Check sheet for the modelled part. Datum: model origin and axes. Units: mm. A direction names the side the tool comes from. Give positions to 0.01 mm unless a question says otherwise; leave off trailing zeros. Write each loop counter-clockwise with the first axis right and the second up, starting at its lowest first coordinate (ties: lowest second). Pieces come first, ordered by that corner, then holes. Notation, with made-up numbers: (-37.75, 50) -> (-14.75, 50) arc R26 cw to (-14.75, 81) -> close; hole circle Ø3 at (-8, 41). An arc over 180 degrees is marked (long way). Answer as a JSON object with one key per item and string values.
from build123d import *

# Parameters (mm, degrees)
BOSS_EXTRU_1_DEPTH                                 = 15
CHAMBRAGE_POUR_VIS_T_TE_HEXAGONALE_M81_D           = 9
CHAMBRAGE_POUR_VIS_T_TE_HEXAGONALE_M81_CBORE_D     = 15
CHAMBRAGE_POUR_VIS_T_TE_HEXAGONALE_M81_CBORE_DEPTH = 8.6
TAP_DRILL_FOR_M5_TAP1_D                            = 4.2
TAP_DRILL_FOR_M5_TAP1_DEPTH                        = 13
TAP_DRILL_FOR_M5_TAP1_TIP                          = 1.2618073
SKETCH25_W                                         = 14
SKETCH25_H                                         = 15
CUT_EXTRUDE6_DEPTH                                 = 16
CONG_1_R                                           = 6
SKETCH11_R                                         = 8.5
CUT_EXTRUDE1_DEPTH                                 = 16
SKETCH12_R                                         = 11
CUT_EXTRUDE2_DEPTH                                 = 11
SKETCH13_W                                         = 24
SKETCH13_H                                         = 24
CUT_EXTRUDE3_DEPTH                                 = 16
FILLET1_R                                          = 6
CUT_EXTRUDE4_DEPTH                                 = 6
FILLET3_R                                          = 14
TAP_DRILL_FOR_M3_TAP1_D                            = 2.5
CHAMFER1_SIZE                                      = 0.5
TAP_DRILL_FOR_M3_TAP2_D                            = 2.5
TAP_DRILL_FOR_M3_TAP3_D                            = 2.5
TROU_POUR_TARAUDAGE_POUR_TROU_TARAUD_M6_D          = 5
TROU_POUR_TARAUDAGE_POUR_TROU_TARAUD_M6_DEPTH      = 20
TROU_POUR_TARAUDAGE_POUR_TROU_TARAUD_M6_TIP        = 1.502151548


with BuildPart() as part:
    # Esquisse1 → Boss.-Extru.1 (new body)
    with BuildSketch(Plane.XY):
        Polygon((-21.072673536, 123.242590707), (54.927326464, 123.242590707), (54.927326464, 18.242590707), (130.927326464, 18.242590707), (130.927326464, -26.757409293), (115.927326464, -26.757409293), (-4.072673536, -146.757409293), (-169.072673536, -146.757409293), (-169.072673536, -76.757409293), (-139.072673536, -46.757409293), (-88.072673536, -46.757409293), (-41.072673536, 0.242590707), (-41.072673536, 103.242590707), align=None)
    extrude(amount=BOSS_EXTRU_1_DEPTH)

    # Chambrage pour vis à tête hexagonale M81 (through all)
    with Locations(Plane(origin=(0, 0, 0), x_dir=(-1, 0, 0), z_dir=(0, 0, -1))):
        with Locations((72.572673536, -78.257409293), (117.572673536, -78.257409293), (72.572673536, -135.257409293), (117.572673536, -135.257409293), (-32.427326464, 85.742590707), (-32.427326464, 40.742590707), (-32.427326464, -4.257409293), (-77.427326464, -4.257409293), (12.572673536, 40.742590707)):
            CounterBoreHole(CHAMBRAGE_POUR_VIS_T_TE_HEXAGONALE_M81_D / 2, CHAMBRAGE_POUR_VIS_T_TE_HEXAGONALE_M81_CBORE_D / 2, CHAMBRAGE_POUR_VIS_T_TE_HEXAGONALE_M81_CBORE_DEPTH)

    # Tap Drill for M5 Tap1
    with Locations(Plane(origin=(0, -146.757409293, 0), x_dir=(-1, 0, 0), z_dir=(0, -1, 0))):
        with Locations((13.072673536, -7.5)):
            Hole(TAP_DRILL_FOR_M5_TAP1_D / 2, depth=TAP_DRILL_FOR_M5_TAP1_DEPTH)
            with Locations((0, 0, -(TAP_DRILL_FOR_M5_TAP1_DEPTH + TAP_DRILL_FOR_M5_TAP1_TIP / 2))):  # 118° drill point
                Cone(0, TAP_DRILL_FOR_M5_TAP1_D / 2, TAP_DRILL_FOR_M5_TAP1_TIP, mode=Mode.SUBTRACT)

    # Sketch25 → Cut-Extrude6 (cut, through all)
    with BuildSketch(Plane(origin=(0, 0, 0), x_dir=(-1, 0, 0), z_dir=(0, 0, -1))):
        with Locations((95.072673536, -54.257409293)):
            Rectangle(SKETCH25_W, SKETCH25_H)
    extrude(amount=-CUT_EXTRUDE6_DEPTH, mode=Mode.SUBTRACT)

    # Congé1
    cong_1_edges = [part.edges().sort_by_distance(p)[0] for p in [
        (-88.072673536, -61.757409293, 7.5),
        (-102.072673536, -46.757409293, 7.5),
        (-102.072673536, -61.757409293, 7.5),
        (54.927326464, 18.242590707, 7.5),
        (130.927326464, 18.242590707, 7.5),
        (130.927326464, -26.757409293, 7.5),
        (115.927326464, -26.757409293, 7.5),
        (-4.072673536, -146.757409293, 7.5),
        (-169.072673536, -76.757409293, 7.5),
        (-139.072673536, -46.757409293, 7.5),
        (-88.072673536, -46.757409293, 7.5),
        (-41.072673536, 0.242590707, 7.5),
        (-41.072673536, 103.242590707, 7.5),
        (-21.072673536, 123.242590707, 7.5),
        (54.927326464, 123.242590707, 7.5),
    ]]
    fillet(cong_1_edges, radius=CONG_1_R)

    # Sketch11 → Cut-Extrude1 (cut, through all)
    with BuildSketch(Plane(origin=(0, 0, 0), x_dir=(-1, 0, 0), z_dir=(0, 0, -1))):
        with Locations((155.072673536, -132.757409293)):
            Circle(SKETCH11_R)
    extrude(amount=-CUT_EXTRUDE1_DEPTH, mode=Mode.SUBTRACT)

    # Sketch12 → Cut-Extrude2 (cut)
    with BuildSketch(Plane(origin=(0, 0, 0), x_dir=(-1, 0, 0), z_dir=(0, 0, -1))):
        with Locations((155.072673536, -132.757409293)):
            Circle(SKETCH12_R)
    extrude(amount=-CUT_EXTRUDE2_DEPTH, mode=Mode.SUBTRACT)

    # Sketch13 → Cut-Extrude3 (cut, through all)
    with BuildSketch(Plane(origin=(0, 0, 0), x_dir=(-1, 0, 0), z_dir=(0, 0, -1))):
        with Locations((48.572673536, -36.757409293)):
            Rectangle(SKETCH13_W, SKETCH13_H)
    extrude(amount=-CUT_EXTRUDE3_DEPTH, mode=Mode.SUBTRACT)

    # Fillet1
    fillet1_edges = [part.edges().sort_by_distance(p)[0] for p in [
        (-36.572673536, -48.757409293, 7.5),
        (-36.572673536, -24.757409293, 7.5),
        (-60.572673536, -24.757409293, 7.5),
        (-60.572673536, -48.757409293, 7.5),
    ]]
    fillet(fillet1_edges, radius=FILLET1_R)

    # Sketch14 → Cut-Extrude4 (cut)
    with BuildSketch(Plane(origin=(0, 0, 0), x_dir=(-1, 0, 0), z_dir=(0, 0, -1))):
        with BuildLine():
            Line((53.794093198, -18.414240629), (59.625660306, -27.52208478))
            ThreePointArc((59.625660306, -27.52208478), (60.33105528, -29.071870895), (60.572673536, -30.757409293))
            Line((60.572673536, -30.757409293), (60.572673536, -42.757409293))
            ThreePointArc((60.572673536, -42.757409293), (60.33105528, -44.442947691), (59.625660306, -45.992733806))
            Line((59.625660306, -45.992733806), (53.794093198, -55.100577956))
            ThreePointArc((53.794093198, -55.100577956), (48.572673536, -57.957409293), (43.351253874, -55.100577956))
            Line((43.351253874, -55.100577956), (37.519686767, -45.992733806))
            ThreePointArc((37.519686767, -45.992733806), (36.814291792, -44.442947691), (36.572673536, -42.757409293))
            Line((36.572673536, -42.757409293), (36.572673536, -30.757409293))
            ThreePointArc((36.572673536, -30.757409293), (36.814291792, -29.071870895), (37.519686767, -27.52208478))
            Line((37.519686767, -27.52208478), (43.351253874, -18.414240629))
            ThreePointArc((43.351253874, -18.414240629), (48.572673536, -15.557409293), (53.794093198, -18.414240629))
        make_face()
    extrude(amount=-CUT_EXTRUDE4_DEPTH, mode=Mode.SUBTRACT)

    # Fillet3
    fillet3_edges = [part.edges().sort_by_distance(p)[0] for p in [
        (-169.072673536, -146.757409293, 7.5),
    ]]
    fillet(fillet3_edges, radius=FILLET3_R)

    # Tap Drill for M3 Tap1 (through all)
    with Locations(Plane(origin=(0, 0, 6), x_dir=(-1, 0, 0), z_dir=(0, 0, -1))):
        with Locations((48.572673536, -21.757409293), (48.572673536, -51.757409293)):
            Hole(TAP_DRILL_FOR_M3_TAP1_D / 2)

    # Chamfer1
    chamfer1_edges = [part.edges().sort_by_distance(p)[0] for p in [
        (-102.072673536, -54.257409293, 0),
        (-95.072673536, -61.757409293, 0),
        (-88.072673536, -52.50004998, 0),
        (-122.330032849, -46.757409293, 0),
        (-64.572673536, -23.257409293, 0),
        (-41.072673536, 51.742590707, 0),
        (-31.072673536, 113.242590707, 0),
        (15.169967151, 123.242590707, 0),
        (54.927326464, 70.742590707, 0),
        (92.927326464, 18.242590707, 0),
        (130.927326464, -4.257409293, 0),
        (121.669967151, -26.757409293, 0),
        (55.927326464, -86.757409293, 0),
        (-169.072673536, -106.00004998, 0),
        (-154.072673536, -61.757409293, 0),
        (53.169967151, 121.485231394, 0),
        (-20.883492756, 122.785867902, 0),
        (-138.883492756, -47.214132098, 0),
        (-168.615950731, -76.946590073, 0),
        (-40.615950731, 103.053409927, 0),
        (129.169967151, 16.485231394, 0),
        (129.169967151, -25.00004998, 0),
        (-4.261854316, -146.300686488, 0),
        (-87.615950731, -46.946590073, 0),
        (-103.830032849, -48.514768606, 0),
        (-100.315314223, -60.00004998, 0),
        (-89.830032849, -60.00004998, 0),
        (116.116507244, -27.214132098, 0),
        (-41.529396341, 0.431771487, 0),
        (56.684685777, 19.99995002, 0),
        (-144.072673536, -132.757409293, 0),
        (-60.572673536, -36.757409293, 0),
        (-36.572673536, -36.757409293, 0),
        (-60.33105528, -44.442947691, 0),
        (-36.814291792, -29.071870895, 0),
        (-60.33105528, -29.071870895, 0),
        (-36.814291792, -44.442947691, 0),
        (-56.709876752, -50.546655881, 0),
        (-40.43547032, -50.546655881, 0),
        (-48.572673536, -57.957409293, 0),
        (-40.43547032, -22.968162704, 0),
        (-56.709876752, -22.968162704, 0),
        (-48.572673536, -15.557409293, 0),
        (-80.815314223, -146.757409293, 0),
        (-164.972168473, -142.656904229, 0),
        (-5.072673536, 40.742590707, 0),
        (84.927326464, -4.257409293, 0),
        (39.927326464, -4.257409293, 0),
        (39.927326464, 40.742590707, 0),
        (39.927326464, 85.742590707, 0),
        (-110.072673536, -135.257409293, 0),
        (-65.072673536, -135.257409293, 0),
        (-110.072673536, -78.257409293, 0),
        (-65.072673536, -78.257409293, 0),
    ]]
    chamfer(chamfer1_edges, length=CHAMFER1_SIZE)

    # Tap Drill for M3 Tap2 (through all)
    with Locations(Plane(origin=(0, 0, 0), x_dir=(-1, 0, 0), z_dir=(0, 0, -1))):
        with Locations((-124.927326464, 12.242590707), (-124.927326464, -20.757409293), (-60.927326464, 12.242590707), (-60.927326464, -20.757409293)):
            Hole(TAP_DRILL_FOR_M3_TAP2_D / 2)

    # Tap Drill for M3 Tap3 (through all)
    with Locations(Plane.XY.offset(15)):
        with Locations((-111.072673536, -52.057409293), (-111.072673536, -62.457409293), (-79.072673536, -62.457409293), (-79.072673536, -52.057409293)):
            Hole(TAP_DRILL_FOR_M3_TAP3_D / 2)

    # Trou pour taraudage pour trou taraudé M61
    with Locations(Plane(origin=(0, -146.757409293, 0), x_dir=(-1, 0, 0), z_dir=(0, -1, 0))):
        with Locations((35.615798493, -7.5), (85.615798493, -7.5)):
            Hole(TROU_POUR_TARAUDAGE_POUR_TROU_TARAUD_M6_D / 2, depth=TROU_POUR_TARAUDAGE_POUR_TROU_TARAUD_M6_DEPTH)
            with Locations((0, 0, -(TROU_POUR_TARAUDAGE_POUR_TROU_TARAUD_M6_DEPTH + TROU_POUR_TARAUDAGE_POUR_TROU_TARAUD_M6_TIP / 2))):  # 118° drill point
                Cone(0, TROU_POUR_TARAUDAGE_POUR_TROU_TARAUD_M6_D / 2, TROU_POUR_TARAUDAGE_POUR_TROU_TARAUD_M6_TIP, mode=Mode.SUBTRACT)


solid = part.part
1. Go/stop test with flat-tipped pins: P1, Ø4.5, axis at y = 54.5, z = 11, coming from the +X side; P2, Ø5, axis at x = 36.5, y = 49, coming from the -Z side; P3, Ø5, axis at x = -33, z = 11, coming from the +Y side; P4, Ø12, axis at x = -72.57, y = -78.26, coming from the -Z side. Record where each tip stops, or that it passes through.
Determined:
{"P1": "x = 54.93", "P2": "z = 0", "P3": "y = 113.82", "P4": "z = 8.6"}
2. Access from +Z, -Z, +X, -X, +Y, -Y to the whole of each face (thin tool, end or side, straight path). Record for faces 1 (the face through (-60.573, -37, 8)), 2 (the face through (-112.045, -73.189, 4.493)), 3 (the face through (-123, -46.757, 8)).
Determined:
{"face 1": "+Z, -Z", "face 2": "-Z", "face 3": "+Z, -Z, -X, +Y"}
3. Mould release check, pull along Y, two halves, no side actions. Record for faces 4 (the face through (-17, -10, 0)), 5 (the face through (-72, -140, 8.6)), 6 (the face through (15, 123.243, 8)), 7 (the face through (-75.889, -75.216, 11.845)): released by +Y, released by -Y, zero draft, split by the parting line, or undercut.
Determined:
{"face 4": "zero draft", "face 5": "undercut", "face 6": "released by +Y", "face 7": "undercut"}
4. Scan lines: L1, parallel to X at y = -81, z = 10.5; L2, parallel to Y at x = -123, z = 7.5; L3, parallel to X at y = 44, z = 10.25. Record each from-to range of solid material in increasing order. Write a range as [from, to].
Determined:
{"L1": "[-169.07, -121.14], [-114.01, -76.14], [-69.01, 61.68]", "L2": "[-146.76, -140.43], [-130.08, -83.43], [-73.08, -46.76]", "L3": "[-41.07, -15.68], [-9.47, 29.32], [35.53, 54.93]"}
5. Sectioned sample at A-A, the plane y = 66. Enter the section's corners in (x, z), plus the area to 3 significant figures.
Determined:
{"outline": "(-41.07, 0.5) -> (-40.57, 0) -> (54.43, 0) -> (54.93, 0.5) -> (54.93, 15) -> (-41.07, 15) -> close", "area": "1,440 mm^2"}
